from build123d import *

# Parameters (mm, degrees)
BOSS_EXTRUDE1_DEPTH   = 25
BOSS_EXTRUDE1_2_DEPTH = 25
BOSS_EXTRUDE2_DEPTH   = 14
SKETCH1_5_W           = 18.467001677
SKETCH1_5_H           = 28
BOSS_EXTRUDE3_DEPTH   = 14
SKETCH2_R             = 12.5
CUT_EXTRUDE1_DEPTH    = 98
CUT_EXTRUDE2_DEPTH    = 98
BOSS_EXTRUDE4_DEPTH   = 15
BOSS_EXTRUDE5_DEPTH   = 15
BOSS_EXTRUDE6_DEPTH   = 30
FILLET1_R             = 5.75
FILLET2_R             = 5.75
FILLET3_R             = 5.75
FILLET4_R             = 5.75
SKETCH9_R             = 12.5
BOSS_EXTRUDE7_DEPTH   = 30


with BuildPart() as part:
    # Sketch1 → Boss-Extrude1 (new, symmetric)
    with BuildSketch(Plane.XY):
        Polygon((5, 13.5), (5, 15), (5, 30), (5, 31.5), (55, 31.5), (55, 13.5), align=None)
    extrude(amount=BOSS_EXTRUDE1_DEPTH, both=True)



with BuildPart() as body_2:
    # Sketch1 → Boss-Extrude1 2 (new, symmetric)
    with BuildSketch(Plane.XY):
        Polygon((5, -13.5), (55, -13.5), (55, -31.5), (5, -31.5), (5, -30), (5, -15), align=None)
    extrude(amount=BOSS_EXTRUDE1_2_DEPTH, both=True)


with BuildPart() as part_1:
    add(part.part)

    add(body_2.part)  # Boss-Extrude2 merges body 2
    # Sketch1_4 → Boss-Extrude2 (add, symmetric)
    with BuildSketch(Plane.XY):
        with BuildLine():
            Line((0, 30), (5, 30))
            Line((5, 30), (5, 15))
            Line((5, 15), (0, 15))
            ThreePointArc((0, 15), (-15, 0), (0, -15))
            Line((0, -15), (5, -15))
            Line((5, -15), (5, -30))
            Line((5, -30), (0, -30))
            ThreePointArc((0, -30), (-15.491933385, -25.690465157), (-26.532998323, -14))
            Line((-26.532998323, -14), (-26.532998323, 14))
            ThreePointArc((-26.532998323, 14), (-15.491933385, 25.690465157), (0, 30))
        make_face()
    extrude(amount=BOSS_EXTRUDE2_DEPTH, both=True)

    # Sketch1_5 → Boss-Extrude3 (add, symmetric)
    with BuildSketch(Plane.XY):
        with Locations((-35.766499162, 0)):
            Rectangle(SKETCH1_5_W, SKETCH1_5_H)
    extrude(amount=BOSS_EXTRUDE3_DEPTH, both=True)

    # Sketch2 → Cut-Extrude1 (cut)
    with BuildSketch(Plane(origin=(0, 31.5, 0), x_dir=(1, 0, 0), z_dir=(0, 1, 0))):
        with Locations(Location((30, 0, 0), (0, 0, 270))):
            Circle(SKETCH2_R)
    extrude(amount=-CUT_EXTRUDE1_DEPTH, mode=Mode.SUBTRACT)

    # Sketch3 → Cut-Extrude2 (cut)
    with BuildSketch(Plane(origin=(0, 31.5, 0), x_dir=(1, 0, 0), z_dir=(0, 1, 0))):
        with BuildLine():
            Line((5, -2.5e-08), (5, -25))
            Line((5, -25), (30, -25))
            ThreePointArc((30, -25), (12.322330479, -17.677669538), (5, -2.5e-08))
        make_face()
        with BuildLine():
            Line((5, 25), (5, -2.5e-08))
            ThreePointArc((5, -2.5e-08), (12.322330462, 17.677669521), (30, 25))
            Line((30, 25), (5, 25))
        make_face()
        with BuildLine():
            ThreePointArc((55, 0), (47.67766953, -17.67766953), (30, -25))
            Line((30, -25), (55, -25))
            Line((55, -25), (55, 0))
        make_face()
        with BuildLine():
            Line((55, 25), (30, 25))
            ThreePointArc((30, 25), (47.67766953, 17.67766953), (55, 0))
            Line((55, 0), (55, 25))
        make_face()
    extrude(amount=-CUT_EXTRUDE2_DEPTH, mode=Mode.SUBTRACT)


with BuildPart() as cut_extrude2_piece_1:
    # of the separate pieces the step leaves, piece 1, a body of its own (cut_extrude2_pieces)
    add(part_1.part.solids().sort_by_distance((5, -30, -14))[0])



with BuildPart() as cut_extrude2_piece_2:
    # of the separate pieces the step leaves, piece 2, a body of its own (cut_extrude2_pieces)
    add(part_1.part.solids().sort_by_distance((5, -13.5, 2.5e-08))[0])


with BuildPart() as cut_extrude2_piece_3:
    # of the separate pieces the step leaves, piece 3, a body of its own (cut_extrude2_pieces)
    add(part_1.part.solids().sort_by_distance((5, 31.5, 2.5e-08))[0])


with BuildPart() as cut_extrude2_piece_1_1:
    add(cut_extrude2_piece_1.part)

    add(cut_extrude2_piece_3.part)  # Boss-Extrude4 merges Cut-Extrude2 piece 3
    # Sketch6 → Boss-Extrude4 (add)
    with BuildSketch(Plane(origin=(0, 30, 0), x_dir=(1, 0, 0), z_dir=(0, 1, 0))):
        with BuildLine():
            Line((9.287684823, 14), (5, 14))
            Line((5, 14), (5, 2.6e-08))
            ThreePointArc((5, 2.6e-08), (6.095943032, 7.320933033), (9.287684823, 14))
        make_face()
        with BuildLine():
            ThreePointArc((9.287684823, -14), (6.095943024, -7.320933008), (5, 2.6e-08))
            Line((5, 2.6e-08), (5, -14))
            Line((5, -14), (9.287684823, -14))
        make_face()
    extrude(amount=-BOSS_EXTRUDE4_DEPTH)


    add(cut_extrude2_piece_2.part)  # Boss-Extrude5 merges Cut-Extrude2 piece 2
    # Sketch7 → Boss-Extrude5 (add)
    with BuildSketch(Plane(origin=(0, -30, 0), x_dir=(-1, 0, 0), z_dir=(0, -1, 0))):
        with BuildLine():
            Line((-5, 0), (-5, 14))
            Line((-5, 14), (-9.287684823, 14))
            ThreePointArc((-9.287684823, 14), (-6.095943028, 7.32093302), (-5, 0))
        make_face()
        with BuildLine():
            Line((-5, -14), (-5, 0))
            ThreePointArc((-5, 0), (-6.095943028, -7.32093302), (-9.287684823, -14))
            Line((-9.287684823, -14), (-5, -14))
        make_face()
    extrude(amount=-BOSS_EXTRUDE5_DEPTH)

    # Sketch8 → Boss-Extrude6 (add)
    with BuildSketch(Plane.ZY.offset(45)):
        Polygon((5.798989873, 14), (-5.798989873, 14), (-14, 5.798989873), (-14, -5.798989873), (-5.798989873, -14), (5.798989873, -14), (14, -5.798989873), (14, 5.798989873), align=None)
    extrude(amount=BOSS_EXTRUDE6_DEPTH)

    # Fillet1
    fillet1_edges = [cut_extrude2_piece_1_1.edges().sort_by_distance(p)[0] for p in [
        (-45, 9.899494937, -9.899494937),
    ]]
    fillet(fillet1_edges, radius=FILLET1_R)

    # Fillet2
    fillet2_edges = [cut_extrude2_piece_1_1.edges().sort_by_distance(p)[0] for p in [
        (-45, 9.899494937, 9.899494937),
    ]]
    fillet(fillet2_edges, radius=FILLET2_R)

    # Fillet3
    fillet3_edges = [cut_extrude2_piece_1_1.edges().sort_by_distance(p)[0] for p in [
        (-45, -9.899494937, -9.899494937),
    ]]
    fillet(fillet3_edges, radius=FILLET3_R)

    # Fillet4
    fillet4_edges = [cut_extrude2_piece_1_1.edges().sort_by_distance(p)[0] for p in [
        (-45, -9.899494937, 9.899494937),
    ]]
    fillet(fillet4_edges, radius=FILLET4_R)

    # Sketch9 → Boss-Extrude7 (add)
    with BuildSketch(Plane.ZY.offset(75)):
        Circle(SKETCH9_R)
    extrude(amount=BOSS_EXTRUDE7_DEPTH)


solid = cut_extrude2_piece_1_1.part
For this review, take the finished solid that the model builds, in its own axes (mm). A direction names the side the tool comes from. Round coordinates to 2 decimals unless told otherwise and drop trailing zeros. Loops run counter-clockwise (first coordinate to the right, second up) from the corner with the lowest first, then second, coordinate; pieces in that order, holes last. Notation, with made-up numbers: (33.25, 22.5) - (78.25, 22.5) arc R21 cw to (78.25, 58.5) - close; hole circle Ø2 at (44.25, 10). An arc over 180 degrees is marked (long way). One line per item, written item: value. Start each with the question number.
Item 1: For L1, parallel to Y at x = 11, z = -11; L2, parallel to Y at x = -9, z = 9; L3, parallel to Z at x = -11.5, y = -26, list the stretches that pass through material, from the lowest coordinate up.
Item 2: The part is to be moulded in two halves that separate along Y. For faces 5 (the cylindrical face through (-89.79, 3.755, 11.923)), 6 (the flat face through (35.9, 13.5, 11.5)), 7 (the flat face through (35.9, -31.5, 11.5)), 8 (the flat face through (-24, 0, 14)), say which applies: +Y half, -Y half, draft (parallel to the pull), parting line (faces both ways), or undercut.
Item 3: Take a section at B-B (y = 24). Give the boundary of the cut face in (x, z), plus the area to 3 significant figures.
Item 4: Take a section at A-A (x = 15). Give the boundary of the cut face in (y, z).
Item 5: For faces 1 (the flat face through (-62.7, -10, 9.8)), 2 (the flat face through (-62.7, 10, -9.8)), 3 (the flat face through (18.5, -13.5, 5.9)), 4 (the flat face through (-75, 0, -13)), list the 3-axis set-ups (+Z, -Z, +X, -X, +Y, -Y) from which the entire face can be reached by the end or side of a thin tool; tool diameter is ignored.
Item 6: Take a section at C-C (z = -3). State how many separate pieces and enclosed holes the cut face has, plus the area to 3 significant figures.
Item 7: Take a section at D-D (y = 0). Give the boundary of the cut face in (x, z).
Item 8: Clearance check with flat-ended pins moving along their axes: pin 1 Ø12 at (y, z) = (12, 6.5) entering from -X; pin 2 Ø2 at (x, y) = (31.5, -24) entering from -Z (3 decimals); pin 3 Ø1.5 at (y, z) = (19.5, -8) entering from -X; pin 4 Ø3 at (y, z) = (1.5, 3.5) entering from +X. State where each tip first meets the part, or that it passes through.
Answer below:
1. L1: y = -31.5 to -13.5, 13.5 to 31.5
1. L2: y = -28.62 to -12, 12 to 28.62
1. L3: z = -14 to 14
2. face 5: parting line
2. face 6: undercut
2. face 7: -Y half
2. face 8: draft
3. outline: (-18, -14) - (9.29, -14) arc R25 ccw (long way) to (9.29, 14) - (-18, 14) - close; hole circle Ø25 at (30, 0)
3. area: 2,160 mm2
4. outline: (-31.5, -20) - (-13.5, -20) - (-13.5, 20) - (-31.5, 20) - close; (13.5, -20) - (31.5, -20) - (31.5, 20) - (13.5, 20) - close
5. face 1: +Z, -X, -Y
5. face 2: -Z, -X, +Y
5. face 3: +Z, -Z, +X
5. face 4: -X
6. separate pieces: 3
6. enclosed holes: 0
6. area: 4,150 mm2
7. outline: (-105, -12.5) - (-75, -12.5) - (-75, -14) - (-15, -14) - (-15, 14) - (-75, 14) - (-75, 12.5) - (-105, 12.5) - close
8. pin 1: stops at x = -105
8. pin 2: stops at z = -24.995
8. pin 3: stops at x = -23.42
8. pin 4: stops at x = -14.7
